Part model, mm, in its own coordinate system. A direction names the side the tool comes from. Coordinates: 2 decimals unless noted, no trailing zeros. Order: outer loops, then holes, each group sorted by start corner. A loop starts at its lowest first (then second) coordinate and runs counter-clockwise, first axis right, second up.
```python
from build123d import *

# Parameters (mm, degrees)
SKETCH1_W           = 30
SKETCH1_H           = 150
BOSS_EXTRUDE1_DEPTH = 3
SKETCH2_W           = 3
SKETCH2_H           = 10
SKETCH2_H_2         = 90
CUT_EXTRUDE1_DEPTH  = 3


with BuildPart() as part:
    # Sketch1 → Boss-Extrude1 (new body)
    with BuildSketch(Plane.XY):
        Rectangle(SKETCH1_W, SKETCH1_H)
    extrude(amount=BOSS_EXTRUDE1_DEPTH)

    # Sketch2 → Cut-Extrude1 (cut)
    with BuildSketch(Plane.XY.offset(3)):
        with Locations((-13.5, 70)):
            Rectangle(SKETCH2_W, SKETCH2_H)
        with Locations((-13.5, -70)):
            Rectangle(SKETCH2_W, SKETCH2_H)
        with Locations((-13.5, 0)):
            Rectangle(SKETCH2_W, SKETCH2_H_2)
    extrude(amount=-CUT_EXTRUDE1_DEPTH, mode=Mode.SUBTRACT)


solid = part.part
```
(1) Drop a flat-ended pin along its axis: pin 1 (0.9 mm diameter, centred on x = -13, z = 1.5, fed in from -Y). Give the stop position or say it passes through.
(2) Pull direction Y, two halves, no side cores. Call faces 1 (the face through (-12, -1, 2)), 2 (the face through (-14, 65, 2)), 3 (the face through (-15, -55, 1)): +Y half, -Y half, draft (parallel to the pull), parting line (faces both ways), or undercut.
(3) Tool access for faces 4 (the face through (-14, 45, 2)), 5 (the face through (-14, -65, 2)), 6 (the face through (-12, 70, 2)): list every direction of +Z, -Z, +X, -X, +Y, -Y with a clear straight run to the whole face (end or side of a thin tool).
(4) Slice it at B-B, the plane y = 8.5. Give the cut face in (x, z).
(5) Probe line 1 (X direction, y = -2, z = 2.2). List the from-to ranges inside material, lowest first.
(6) Slice it at A-A, the plane z = 2.5. Give the cut face in (x, y).
Here are the results:
1. pin 1: stops at y = -65
2. face 1: undercut
2. face 2: +Y half
2. face 3: draft
3. face 4: +Z, -Z, -X
3. face 5: +Z, -Z, -X, -Y
3. face 6: +Z, -Z, -X, +Y
4. outline: (-12, 0) - (15, 0) - (15, 3) - (-12, 3) - close
5. line 1: x = -12 to 15
6. outline: (-15, -65) - (-12, -65) - (-12, -75) - (15, -75) - (15, 75) - (-12, 75) - (-12, 65) - (-15, 65) - (-15, 45) - (-12, 45) - (-12, -45) - (-15, -45) - close
